Geometry: final body of the model. Coordinates: model frame, mm. Face numbers are marked on the shaded views. A direction names the side the tool comes from. Coordinates: 2 decimals unless noted, no trailing zeros. Loops run counter-clockwise (first coordinate to the right, second up) from the corner with the lowest first, then second, coordinate; pieces in that order, holes last. Notation, with made-up numbers: (63, 18.5) - (114, 18.5) arc R24 ccw to (114, 37.5) - close; hole circle Ø6 at (77.25, -1.5). An arc over 180 degrees is marked (long way). Put each result on its own line as item: value. Start each with the question number.
1) Section C-C on x = 64. Output: boundary loops of the cut face in (y, z), and give its area (3 significant figures).
2) Section A-A on z = -15. Output: boundary loops of the cut face in (x, y), and give its area (3 significant figures).
3) Material intervals for line 1 along Z through (x, y) = (0, -21); line 2 along X through (y, z) = (5, 0); line 3 along Y through (x, z) = (-63, 127), sorted ascending. Write a range as from..to.
4) Section D-D on z = 63.5. Output: boundary loops of the cut face in (x, y), and give its area (3 significant figures).
5) Section B-B on y = 33. Output: boundary loops of the cut face in (x, z), and give its area (3 significant figures).
6) Reachability of the marked faces 1 and 2 from +Z, -Z, +X, -X, +Y, -Y: full face, straight path, thin tool, end or side. Return the list, or none.
7) Contact query for flat-ended pins moving along their axis: pin 1 Ø8 at (x, y) = (-4.5, 64.5) entering from +Z; pin 2 Ø15 at (x, z) = (1.5, 19.5) entering from -Y; pin 3 Ø8 at (x, z) = (158.5, -124) entering from -Y. Output: stop coordinate, or through.
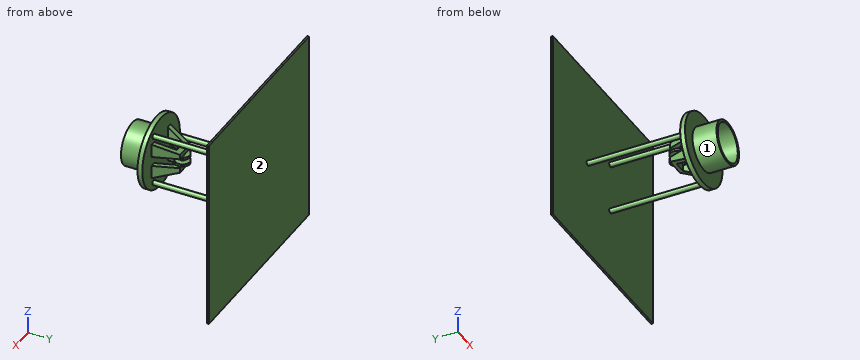
```python
from build123d import *

# Parameters (mm, degrees)
SKETCH1_R               = 75
BOSS_EXTRUDE1_DEPTH     = 10
SKETCH2_R               = 45
SKETCH2_R_2             = 40
BOSS_EXTRUDE2_DEPTH     = 50
SKETCH5_W               = 75
SKETCH5_H               = 75
BOSS_EXTRUDE3_DEPTH     = 50
CUT_EXTRUDE2_DEPTH      = 103
CUT_EXTRUDE3_DEPTH      = 103
CUT_EXTRUDE3_DEPTH_BACK = 103
SKETCH9_W               = 20
SKETCH9_H               = 50
CUT_EXTRUDE4_DEPTH      = 103
CUT_EXTRUDE4_DEPTH_BACK = 103
SKETCH10_R              = 5
CUT_EXTRUDE5_DEPTH      = 103
SKETCH11_R              = 5
SKETCH13_W              = 400
SKETCH13_H              = 400
BOSS_EXTRUDE4_DEPTH     = 4


with BuildPart() as part:
    # Sketch1 → Boss-Extrude1 (new body)
    with BuildSketch(Plane(origin=(0, 0, 0), x_dir=(1, 0, 0), z_dir=(0, 1, 0))):
        Circle(SKETCH1_R)
    extrude(amount=BOSS_EXTRUDE1_DEPTH)

    # Sketch2 → Boss-Extrude2 (add)
    with BuildSketch(Plane.XZ):
        Circle(SKETCH2_R)
        Circle(SKETCH2_R_2, mode=Mode.SUBTRACT)
    extrude(amount=BOSS_EXTRUDE2_DEPTH)

    # Sketch5 → Boss-Extrude3 (add)
    with BuildSketch(Plane(origin=(0, 10, 0), x_dir=(1, 0, 0), z_dir=(0, 1, 0))):
        Rectangle(SKETCH5_W, SKETCH5_H)
    extrude(amount=BOSS_EXTRUDE3_DEPTH)

    # Sketch6 → Cut-Extrude2 (cut)
    with BuildSketch(Plane.XY.offset(37.5)):
        Polygon((20, 60), (37.5, 10), (43.069722315, 10), (43.069722315, 63.034625831), (-42.678571429, 63.034625831), (-42.678571429, 10), (-37.5, 10), (-20, 60), align=None)
        Polygon((-12.90518995, 50), (-26.90518995, 10), (26.90518995, 10), (12.90518995, 50), align=None)
    extrude(amount=-CUT_EXTRUDE2_DEPTH, mode=Mode.SUBTRACT)

    # Sketch7 → Cut-Extrude3 (cut, two sides)
    with BuildSketch(Plane(origin=(0, 0, 0), x_dir=(0, 0, -1), z_dir=(1, 0, 0))) as cut_extrude3_sk:
        Polygon((20, 60), (-20, 60), (-37.5, 10), (-47.69302584, 10), (-47.69302584, 63.764621125), (47.449694076, 63.764621125), (47.449694076, 10), (37.5, 10), align=None)
    extrude(amount=CUT_EXTRUDE3_DEPTH, mode=Mode.SUBTRACT)
    extrude(cut_extrude3_sk.sketch, amount=-CUT_EXTRUDE3_DEPTH_BACK, mode=Mode.SUBTRACT)

    # Sketch9 → Cut-Extrude4 (cut, two sides)
    with BuildSketch(Plane(origin=(0, 0, 0), x_dir=(0, 0, -1), z_dir=(1, 0, 0))) as cut_extrude4_sk:
        with Locations((0, 35)):
            Rectangle(SKETCH9_W, SKETCH9_H)
    extrude(amount=CUT_EXTRUDE4_DEPTH, mode=Mode.SUBTRACT)
    extrude(cut_extrude4_sk.sketch, amount=-CUT_EXTRUDE4_DEPTH_BACK, mode=Mode.SUBTRACT)

    # Sketch10 → Cut-Extrude5 (cut)
    with BuildSketch(Plane(origin=(0, 10, 0), x_dir=(1, 0, 0), z_dir=(0, 1, 0))):
        Circle(SKETCH10_R)
    extrude(amount=-CUT_EXTRUDE5_DEPTH, mode=Mode.SUBTRACT)

    # Sweep1: sweep along a curve in space
    with BuildLine() as sweep1_path:
        Line((-60, 10, 0), (-60, 210, 0))
    # Sketch11 → Sweep1 (sweep)
    with BuildSketch(Plane(origin=(0, 10, 0), x_dir=(1, 0, 0), z_dir=(0, 1, 0))):
        with Locations((-60, 0)):
            Circle(SKETCH11_R)
        with Locations((30, 51.961524227)):
            Circle(SKETCH11_R)
        with Locations((30, -51.961524227)):
            Circle(SKETCH11_R)
    sweep(path=sweep1_path.line)

    # Sketch13 → Boss-Extrude4 (add)
    with BuildSketch(Plane(origin=(0, 210, 0), x_dir=(1, 0, 0), z_dir=(0, 1, 0))):
        Rectangle(SKETCH13_W, SKETCH13_H)
    extrude(amount=BOSS_EXTRUDE4_DEPTH)

    # Sketch17 → Revolve2 (revolve)
    with BuildSketch(Plane(origin=(0, 0, 0), x_dir=(0, 0, -1), z_dir=(1, 0, 0))):
        Polygon((10, 55), (10, 70), (5, 70), (3.237517532, 60.004465223), (-3.237517532, 60.004465223), (-5, 70), (-10, 70), (-10, 55), align=None)
    revolve(axis=Axis((0, 55, -10), (0, 0, 1)))


solid = part.part
```
Answer block:
1. outline: (0, -39.1) - (10, -39.1) - (10, 39.1) - (0, 39.1) - close; (210, -200) - (214, -200) - (214, 200) - (210, 200) - close
1. area: 2,380 mm²
2. outline: (-200, 210) - (200, 210) - (200, 214) - (-200, 214) - close; (-73.48, 0) - (-42.43, 0) - (-42.43, -50) - (-37.08, -50) - (-37.08, 0) - (37.08, 0) - (37.08, -50) - (42.43, -50) - (42.43, 0) - (73.48, 0) - (73.48, 10) - (37.5, 10) - (20, 60) - (-20, 60) - (-37.5, 10) - (-73.48, 10) - close; hole (-26.91, 10) - (26.91, 10) - (12.91, 50) - (-12.91, 50) - close
2. area: 4,890 mm²
3. line 1: z = -45..-40, 40..45
3. line 2: x = -75..-5, 5..75
3. line 3: y = 210..214
4. outline: (-200, 210) - (200, 210) - (200, 214) - (-200, 214) - close; (-39.91, 0) - (39.91, 0) - (39.91, 10) - (-39.91, 10) - close
4. area: 2,400 mm²
5. outline: circle Ø10 at (-60, 0); (-29.45, -29.45) - (-18.86, -29.45) - (-18.86, -10) - (-29.45, -10) - close; (-29.45, 10) - (-18.86, 10) - (-18.86, 29.45) - (-29.45, 29.45) - close; (18.86, -29.45) - (29.45, -29.45) - (29.45, -10) - (18.86, -10) - close; (18.86, 10) - (29.45, 10) - (29.45, 29.45) - (18.86, 29.45) - close; circle Ø10 at (30, -51.96); circle Ø10 at (30, 51.96)
5. area: 1,060 mm²
6. face 1: -Y
6. face 2: +Z, -Z, +X, -X, +Y
7. pin 1: stops at z = 10
7. pin 2: stops at y = 0
7. pin 3: stops at y = 210
